For this review, take the finished solid that the model builds, in its own axes (mm). Round coordinates to 2 decimals unless told otherwise and drop trailing zeros. Order: outer loops, then holes, each group sorted by start corner. A loop starts at its lowest first (then second) coordinate and runs counter-clockwise, first axis right, second up. Notation, with made-up numbers: M -18,-13 L 38,-13 A18 cw 38,17 Z; hole C 12.25,9.25 d7. An arc over 180 degrees is marked long. Use a Markdown table: item, result.
from build123d import *

# Parameters (mm, degrees)
SKETCH1_W               = 3
SKETCH1_H               = 49.4545
SKETCH1_W_2             = 20.4615
SKETCH1_H_2             = 3
SKETCH1_H_3             = 27.7273
SKETCH1_W_3             = 162
SKETCH1_H_4             = 261
SKETCH1_W_4             = 20
BOSS_EXTRUDE1_DEPTH     = 3
SKETCH2_W               = 10.5
SKETCH2_H               = 3.2
SKETCH2_W_2             = 2.5
SKETCH2_H_2             = 5.2
CUT_EXTRUDE1_DEPTH      = 10
SKETCH3_W               = 35
SKETCH3_H               = 25
SKETCH3_W_2             = 30
SKETCH3_H_2             = 50
CUT_EXTRUDE2_DEPTH      = 1
CUT_EXTRUDE2_DEPTH_BACK = 4
SKETCH4_W               = 162
SKETCH4_H               = 25
BOSS_EXTRUDE2_DEPTH     = 3
FILLET1_R               = 2


with BuildPart() as part:
    # Sketch1 → Boss-Extrude1 (new body)
    with BuildSketch(Plane(origin=(0, 0, 0), x_dir=(1, 0, 0), z_dir=(0, 1, 0))):
        Polygon((-133, -152.5), (-133, -155.5), (133, -155.5), (133, -152.5), (123, -152.5), (123, -149.5), (133, -149.5), (133, -27.7273), (105, -27.7273), (105, -15.2273), (108, -15.2273), (108, -5.2273), (105, -5.2273), (105, 35.4545), (108, 35.4545), (108, 45.4545), (105, 45.4545), (105, 55.4545), (127, 55.4545), (127, 69.3181), (133, 69.3181), (133, 155.5), (-133, 155.5), (-133, 69.3181), (-127, 69.3181), (-127, 55.4545), (-105, 55.4545), (-105, 45.4545), (-108, 45.4545), (-108, 35.4545), (-105, 35.4545), (-105, -5.2273), (-108, -5.2273), (-108, -15.2273), (-105, -15.2273), (-105, -27.7273), (-133, -27.7273), (-133, -149.5), (-123, -149.5), (-123, -152.5), align=None)
        with Locations((-128.5, -121.77275)):
            Rectangle(SKETCH1_W, SKETCH1_H, mode=Mode.SUBTRACT)
        with Locations((-81.846, -151)):
            Rectangle(SKETCH1_W_2, SKETCH1_H_2, mode=Mode.SUBTRACT)
        with Locations((-40.923, -151)):
            Rectangle(SKETCH1_W_2, SKETCH1_H_2, mode=Mode.SUBTRACT)
        with Locations((0, -151)):
            Rectangle(SKETCH1_W_2, SKETCH1_H_2, mode=Mode.SUBTRACT)
        with Locations((-128.5, -55.45455)):
            Rectangle(SKETCH1_W, SKETCH1_H_3, mode=Mode.SUBTRACT)
        with Locations((40.923, -151)):
            Rectangle(SKETCH1_W_2, SKETCH1_H_2, mode=Mode.SUBTRACT)
        with Locations((81.846, -151)):
            Rectangle(SKETCH1_W_2, SKETCH1_H_2, mode=Mode.SUBTRACT)
        with Locations((128.5, -121.77275)):
            Rectangle(SKETCH1_W, SKETCH1_H, mode=Mode.SUBTRACT)
        with Locations((128.5, -55.45455)):
            Rectangle(SKETCH1_W, SKETCH1_H_3, mode=Mode.SUBTRACT)
        Rectangle(SKETCH1_W_3, SKETCH1_H_4, mode=Mode.SUBTRACT)
        with Locations((-128.5, 110.90905)):
            Rectangle(SKETCH1_W, SKETCH1_H_3, mode=Mode.SUBTRACT)
        with Locations((-100, 151)):
            Rectangle(SKETCH1_W_4, SKETCH1_H_2, mode=Mode.SUBTRACT)
        with Locations((-60, 151)):
            Rectangle(SKETCH1_W_4, SKETCH1_H_2, mode=Mode.SUBTRACT)
        with Locations((-20, 151)):
            Rectangle(SKETCH1_W_4, SKETCH1_H_2, mode=Mode.SUBTRACT)
        with Locations((20, 151)):
            Rectangle(SKETCH1_W_4, SKETCH1_H_2, mode=Mode.SUBTRACT)
        with Locations((60, 151)):
            Rectangle(SKETCH1_W_4, SKETCH1_H_2, mode=Mode.SUBTRACT)
        with Locations((128.5, 110.90905)):
            Rectangle(SKETCH1_W, SKETCH1_H_3, mode=Mode.SUBTRACT)
        with Locations((100, 151)):
            Rectangle(SKETCH1_W_4, SKETCH1_H_2, mode=Mode.SUBTRACT)
    extrude(amount=BOSS_EXTRUDE1_DEPTH)

    # Sketch2 → Cut-Extrude1 (cut)
    with BuildSketch(Plane(origin=(0, 3, 0), x_dir=(1, 0, 0), z_dir=(0, 1, 0))):
        with Locations((-102.75, -10.2273)):
            Rectangle(SKETCH2_W, SKETCH2_H)
        with Locations((102.75, -10.2273)):
            Rectangle(SKETCH2_W, SKETCH2_H)
        with Locations((103.575, -10.2273)):
            Rectangle(SKETCH2_W_2, SKETCH2_H_2)
        with Locations((-103.575, -10.2273)):
            Rectangle(SKETCH2_W_2, SKETCH2_H_2)
    extrude(amount=-CUT_EXTRUDE1_DEPTH, mode=Mode.SUBTRACT)

    # Sketch3 → Cut-Extrude2 (cut, two sides)
    with BuildSketch(Plane(origin=(0, 3, 0), x_dir=(1, 0, 0), z_dir=(0, 1, 0))) as cut_extrude2_sk:
        with Locations((0, -143)):
            Rectangle(SKETCH3_W, SKETCH3_H)
        with Locations((-96, -92.3182)):
            Rectangle(SKETCH3_W_2, SKETCH3_H_2)
        with Locations((96, -92.3182)):
            Rectangle(SKETCH3_W_2, SKETCH3_H_2)
    extrude(amount=CUT_EXTRUDE2_DEPTH, mode=Mode.SUBTRACT)
    extrude(cut_extrude2_sk.sketch, amount=-CUT_EXTRUDE2_DEPTH_BACK, mode=Mode.SUBTRACT)

    # Sketch4 → Boss-Extrude2 (add)
    with BuildSketch(Plane.XZ):
        with Locations((0, 54.8182)):
            Rectangle(SKETCH4_W, SKETCH4_H)
    extrude(amount=-BOSS_EXTRUDE2_DEPTH)

    # Fillet1
    fillet1_edges = [part.edges().sort_by_distance(p)[0] for p in [
        (-133, 1.5, -155.5),
        (133, 1.5, -155.5),
        (133, 1.5, 155.5),
        (-133, 1.5, 155.5),
        (81, 1.5, -130.5),
        (-81, 1.5, -130.5),
        (-81, 1.5, 130.5),
        (81, 1.5, 130.5),
        (17.5, 1.5, 130.5),
        (17.5, 1.5, 155.5),
        (-17.5, 1.5, 155.5),
        (-17.5, 1.5, 130.5),
        (-111, 1.5, 117.3182),
        (-111, 1.5, 67.3182),
        (81, 1.5, 117.3182),
        (111, 1.5, 67.3182),
        (111, 1.5, 117.3182),
        (-81, 1.5, 42.3182),
        (81, 1.5, 42.3182),
    ]]
    fillet(fillet1_edges, radius=FILLET1_R)


solid = part.part
Q1. Add section A-A (z = -90). Write out the cut boundary in (x, y), then the cut area to 3 significant figures.
Determined:
| item | result |
|---|---|
| outline | M -133,0 L -81,0 L -81,3 L -133,3 Z; M 81,0 L 133,0 L 133,3 L 81,3 Z |
| area | 312 mm^2 |
Q2. Add section D-D (y = 1.7). Give the number of separate pieces and of enclosed holes in the cut face, then the cut area to 3 significant figures.
Determined:
| item | result |
|---|---|
| separate pieces | 1 |
| enclosed holes | 17 |
| area | 34,500 mm^2 |
Q3. Wall thickness on line 1 along Z through (x, y) = (-39, 1.75); line 2 along X through (y, z) = (0.95, 69); line 3 along Z through (x, y) = (-60, 1.6): over which ranges is each line inside the solid? List them lowest first. Write a range as [from, to].
Determined:
| item | result |
|---|---|
| line 1 | z = [-155.5, -130.5], [42.32, 67.32], [130.5, 149.5], [152.5, 155.5] |
| line 2 | x = [-133, -130], [-127, -110.97], [110.97, 127], [130, 133] |
| line 3 | z = [-155.5, -152.5], [-149.5, -130.5], [42.32, 67.32], [130.5, 155.5] |
Q4. Clearance check with flat-ended pins moving along their axes: pin 1 (1.5 mm diameter, centred on y = 2, z = 151.5, fed in from -X); pin 2 (0.9 mm diameter, centred on y = 1.5, z = 6, fed in from -X); pin 3 (0.9 mm diameter, centred on y = 1, z = -40.5, fed in from +X). State where each tip first meets the part, or that it passes through.
Determined:
| item | result |
|---|---|
| pin 1 | stops at x = -123 |
| pin 2 | stops at x = -108 |
| pin 3 | stops at x = 108 |
Q5. Add section C-C (z = 50). Write out the cut boundary in (x, y).
Determined:
| item | result |
|---|---|
| outline | M -133,0 L -130,0 L -130,3 L -133,3 Z; M -127,0 L 127,0 L 127,3 L -127,3 Z; M 130,0 L 133,0 L 133,3 L 130,3 Z |
Q6. Add section B-B (x = -57.5). Write out the cut boundary in (y, z), then the cut area to 3 significant figures.
Determined:
| item | result |
|---|---|
| outline | M 0,-155.5 L 3,-155.5 L 3,-152.5 L 0,-152.5 Z; M 0,-149.5 L 3,-149.5 L 3,-130.5 L 0,-130.5 Z; M 0,42.32 L 3,42.32 L 3,67.32 L 0,67.32 Z; M 0,130.5 L 3,130.5 L 3,155.5 L 0,155.5 Z |
| area | 216 mm^2 |
